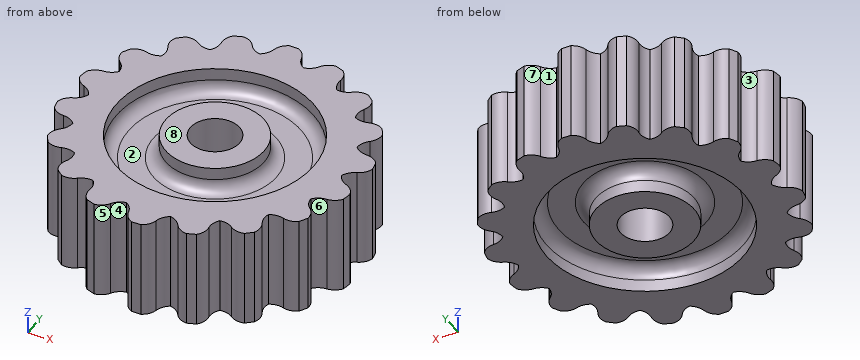
from build123d import *

# Parameters (mm, degrees)
CUT_EXTRUDE4_DEPTH      = 60.56828015
CUT_EXTRUDE4_DEPTH_BACK = 60.56828015


with BuildPart() as part:
    # Sketch1 → Revolve1 (revolve)
    with BuildSketch(Plane(origin=(0, 0, 0), x_dir=(0, 0, -1), z_dir=(1, 0, 0)), mode=Mode.PRIVATE) as revolve1_sk:
        with BuildLine():
            ThreePointArc((9.525, 25.4), (7.27993597, 24.47006403), (6.35, 22.225))
            Line((6.35, 22.225), (6.35, 15.875))
            ThreePointArc((6.35, 15.875), (7.27993597, 13.62993597), (9.525, 12.7))
            Line((9.525, 12.7), (12.7, 12.7))
            Line((12.7, 12.7), (12.7, 6.35))
            Line((12.7, 6.35), (-12.7, 6.35))
            Line((-12.7, 6.35), (-12.7, 12.7))
            Line((-12.7, 12.7), (-9.525, 12.7))
            ThreePointArc((-9.525, 12.7), (-7.27993597, 13.62993597), (-6.35, 15.875))
            Line((-6.35, 15.875), (-6.35, 22.225))
            ThreePointArc((-6.35, 22.225), (-7.27993597, 24.47006403), (-9.525, 25.4))
            Line((-9.525, 25.4), (-12.7, 25.4))
            Line((-12.7, 25.4), (-12.7, 38.1))
            Line((-12.7, 38.1), (12.7, 38.1))
            Line((12.7, 38.1), (12.7, 25.4))
            Line((12.7, 25.4), (9.525, 25.4))
        make_face()
    revolve(revolve1_sk.sketch.rotate(Axis((0, 0, 45.501840491), (0, 0, -1)), 90), axis=Axis((0, 0, 45.501840491), (0, 0, -1)))

    # Sketch2 → Cut-Extrude4 (cut, two sides: drawn at the far end of the back side and taken through both)
    with BuildSketch(Plane.XY.offset(12.7).offset(-CUT_EXTRUDE4_DEPTH_BACK)):
        with BuildLine():
            ThreePointArc((35.210604435, 2.593640551), (33.661156199, 1.568112092), (32.6644, 0))
            ThreePointArc((32.6644, 0), (33.661156199, -1.568112092), (35.210604435, -2.593640551))
            ThreePointArc((35.210604435, -2.593640551), (36.804464445, -3.712859333), (37.710053333, -5.437083557))
            ThreePointArc((37.710053333, -5.437083557), (38.1, 0), (37.710053333, 5.437083557))
            ThreePointArc((37.710053333, 5.437083557), (36.804464445, 3.712859333), (35.210604435, 2.593640551))
        make_face()
        with BuildLine():
            ThreePointArc((32.200067848, 14.479960862), (31.094814165, 12.98633683), (30.694495642, 11.17188277))
            ThreePointArc((30.694495642, 11.17188277), (32.16746601, 10.039250106), (33.974222474, 9.605511089))
            ThreePointArc((33.974222474, 9.605511089), (35.854756332, 9.098921688), (37.295450944, 7.788410548))
            ThreePointArc((37.295450944, 7.788410548), (35.802288852, 13.030967461), (33.576266749, 18.006785143))
            ThreePointArc((33.576266749, 18.006785143), (33.31501097, 16.076814721), (32.200067848, 14.479960862))
        make_face()
        with BuildLine():
            ThreePointArc((33.974222474, -9.605511089), (32.16746601, -10.039250106), (30.694495642, -11.17188277))
            ThreePointArc((30.694495642, -11.17188277), (31.094814165, -12.98633683), (32.200067848, -14.479960862))
            ThreePointArc((32.200067848, -14.479960862), (33.31501097, -16.076814721), (33.576266749, -18.006785143))
            ThreePointArc((33.576266749, -18.006785143), (35.802288852, -13.030967461), (37.295450944, -7.788410548))
            ThreePointArc((37.295450944, -7.788410548), (35.854756332, -9.098921688), (33.974222474, -9.605511089))
        make_face()
        with BuildLine():
            ThreePointArc((25.305727856, 24.619784192), (24.777978632, 22.838217687), (25.022382108, 20.996271598))
            ThreePointArc((25.022382108, 20.996271598), (26.793904679, 20.435730578), (28.640047877, 20.646096329))
            ThreePointArc((28.640047877, 20.646096329), (30.580435445, 20.813238467), (32.382466749, 20.074507397))
            ThreePointArc((32.382466749, 20.074507397), (29.186293283, 24.490207929), (25.392686862, 28.404602689))
            ThreePointArc((25.392686862, 28.404602689), (25.807275495, 26.501668986), (25.305727856, 24.619784192))
        make_face()
        with BuildLine():
            ThreePointArc((28.640047877, -20.646096329), (26.793904679, -20.435730578), (25.022382108, -20.996271598))
            ThreePointArc((25.022382108, -20.996271598), (24.777978632, -22.838217687), (25.305727856, -24.619784192))
            ThreePointArc((25.305727856, -24.619784192), (25.807275495, -26.501668986), (25.392686862, -28.404602689))
            ThreePointArc((25.392686862, -28.404602689), (29.186293283, -24.490207929), (32.382466749, -20.074507397))
            ThreePointArc((32.382466749, -20.074507397), (30.580435445, -20.813238467), (28.640047877, -20.646096329))
        make_face()
        with BuildLine():
            ThreePointArc((15.359143612, 31.790098199), (15.472553192, 29.935472436), (16.3322, 28.288200199))
            ThreePointArc((16.3322, 28.288200199), (18.188603008, 28.367360343), (19.851460823, 29.196457648))
            ThreePointArc((19.851460823, 29.196457648), (21.617662725, 30.017171516), (23.56367915, 29.939322386))
            ThreePointArc((23.56367915, 29.939322386), (19.05, 32.995567884), (14.146374183, 35.376405943))
            ThreePointArc((14.146374183, 35.376405943), (15.18680172, 33.730030848), (15.359143612, 31.790098199))
        make_face()
        with BuildLine():
            ThreePointArc((19.851460823, -29.196457648), (18.188603008, -28.367360343), (16.3322, -28.288200199))
            ThreePointArc((16.3322, -28.288200199), (15.472553192, -29.935472436), (15.359143612, -31.790098199))
            ThreePointArc((15.359143612, -31.790098199), (15.18680172, -33.730030848), (14.146374183, -35.376405943))
            ThreePointArc((14.146374183, -35.376405943), (19.05, -32.995567884), (23.56367915, -29.939322386))
            ThreePointArc((23.56367915, -29.939322386), (21.617662725, -30.017171516), (19.851460823, -29.196457648))
        make_face()
        with BuildLine():
            ThreePointArc((3.560019972, 35.126057191), (4.300909486, 33.422067408), (5.672113535, 32.168154367))
            ThreePointArc((5.672113535, 32.168154367), (7.389487378, 32.877467793), (8.668494618, 34.225295281))
            ThreePointArc((8.668494618, 34.225295281), (10.047480837, 35.600590674), (11.902764082, 36.193013237))
            ThreePointArc((11.902764082, 36.193013237), (6.615995569, 37.52117539), (1.1938, 38.081292541))
            ThreePointArc((1.1938, 38.081292541), (2.734575524, 36.890053188), (3.560019972, 35.126057191))
        make_face()
        with BuildLine():
            ThreePointArc((8.668494618, -34.225295281), (7.389487378, -32.877467793), (5.672113535, -32.168154367))
            ThreePointArc((5.672113535, -32.168154367), (4.300909486, -33.422067408), (3.560019972, -35.126057191))
            ThreePointArc((3.560019972, -35.126057191), (2.734575524, -36.890053188), (1.1938, -38.081292541))
            ThreePointArc((1.1938, -38.081292541), (6.615995569, -37.52117539), (11.902764082, -36.193013237))
            ThreePointArc((11.902764082, -36.193013237), (10.047480837, -35.600590674), (8.668494618, -34.225295281))
        make_face()
        with BuildLine():
            ThreePointArc((-8.668494618, 34.225295281), (-7.389487378, 32.877467793), (-5.672113535, 32.168154367))
            ThreePointArc((-5.672113535, 32.168154367), (-4.300909486, 33.422067408), (-3.560019972, 35.126057191))
            ThreePointArc((-3.560019972, 35.126057191), (-2.734575524, 36.890053188), (-1.1938, 38.081292541))
            ThreePointArc((-1.1938, 38.081292541), (-6.615995569, 37.52117539), (-11.902764082, 36.193013237))
            ThreePointArc((-11.902764082, 36.193013237), (-10.047480837, 35.600590674), (-8.668494618, 34.225295281))
        make_face()
        with BuildLine():
            ThreePointArc((-3.560019972, -35.126057191), (-4.300909486, -33.422067408), (-5.672113535, -32.168154367))
            ThreePointArc((-5.672113535, -32.168154367), (-7.389487378, -32.877467793), (-8.668494618, -34.225295281))
            ThreePointArc((-8.668494618, -34.225295281), (-10.047480837, -35.600590674), (-11.902764082, -36.193013237))
            ThreePointArc((-11.902764082, -36.193013237), (-6.615995569, -37.52117539), (-1.1938, -38.081292541))
            ThreePointArc((-1.1938, -38.081292541), (-2.734575524, -36.890053188), (-3.560019972, -35.126057191))
        make_face()
        with BuildLine():
            ThreePointArc((-19.851460823, 29.196457648), (-18.188603008, 28.367360343), (-16.3322, 28.288200199))
            ThreePointArc((-16.3322, 28.288200199), (-15.472553192, 29.935472436), (-15.359143612, 31.790098199))
            ThreePointArc((-15.359143612, 31.790098199), (-15.18680172, 33.730030848), (-14.146374183, 35.376405943))
            ThreePointArc((-14.146374183, 35.376405943), (-19.05, 32.995567884), (-23.56367915, 29.939322386))
            ThreePointArc((-23.56367915, 29.939322386), (-21.617662725, 30.017171516), (-19.851460823, 29.196457648))
        make_face()
        with BuildLine():
            ThreePointArc((-15.359143612, -31.790098199), (-15.472553192, -29.935472436), (-16.3322, -28.288200199))
            ThreePointArc((-16.3322, -28.288200199), (-18.188603008, -28.367360343), (-19.851460823, -29.196457648))
            ThreePointArc((-19.851460823, -29.196457648), (-21.617662725, -30.017171516), (-23.56367915, -29.939322386))
            ThreePointArc((-23.56367915, -29.939322386), (-19.05, -32.995567884), (-14.146374183, -35.376405943))
            ThreePointArc((-14.146374183, -35.376405943), (-15.18680172, -33.730030848), (-15.359143612, -31.790098199))
        make_face()
        with BuildLine():
            ThreePointArc((-28.640047877, 20.646096329), (-26.793904679, 20.435730578), (-25.022382108, 20.996271598))
            ThreePointArc((-25.022382108, 20.996271598), (-24.777978632, 22.838217687), (-25.305727856, 24.619784192))
            ThreePointArc((-25.305727856, 24.619784192), (-25.807275495, 26.501668986), (-25.392686862, 28.404602689))
            ThreePointArc((-25.392686862, 28.404602689), (-29.186293283, 24.490207929), (-32.382466749, 20.074507397))
            ThreePointArc((-32.382466749, 20.074507397), (-30.580435445, 20.813238467), (-28.640047877, 20.646096329))
        make_face()
        with BuildLine():
            ThreePointArc((-25.305727856, -24.619784192), (-24.777978632, -22.838217687), (-25.022382108, -20.996271598))
            ThreePointArc((-25.022382108, -20.996271598), (-26.793904679, -20.435730578), (-28.640047877, -20.646096329))
            ThreePointArc((-28.640047877, -20.646096329), (-30.580435445, -20.813238467), (-32.382466749, -20.074507397))
            ThreePointArc((-32.382466749, -20.074507397), (-29.186293283, -24.490207929), (-25.392686862, -28.404602689))
            ThreePointArc((-25.392686862, -28.404602689), (-25.807275495, -26.501668986), (-25.305727856, -24.619784192))
        make_face()
        with BuildLine():
            ThreePointArc((-33.974222474, 9.605511089), (-32.16746601, 10.039250106), (-30.694495642, 11.17188277))
            ThreePointArc((-30.694495642, 11.17188277), (-31.094814165, 12.98633683), (-32.200067848, 14.479960862))
            ThreePointArc((-32.200067848, 14.479960862), (-33.31501097, 16.076814721), (-33.576266749, 18.006785143))
            ThreePointArc((-33.576266749, 18.006785143), (-35.802288852, 13.030967461), (-37.295450944, 7.788410548))
            ThreePointArc((-37.295450944, 7.788410548), (-35.854756332, 9.098921688), (-33.974222474, 9.605511089))
        make_face()
        with BuildLine():
            ThreePointArc((-32.200067848, -14.479960862), (-31.094814165, -12.98633683), (-30.694495642, -11.17188277))
            ThreePointArc((-30.694495642, -11.17188277), (-32.16746601, -10.039250106), (-33.974222474, -9.605511089))
            ThreePointArc((-33.974222474, -9.605511089), (-35.854756332, -9.098921688), (-37.295450944, -7.788410548))
            ThreePointArc((-37.295450944, -7.788410548), (-35.802288852, -13.030967461), (-33.576266749, -18.006785143))
            ThreePointArc((-33.576266749, -18.006785143), (-33.31501097, -16.076814721), (-32.200067848, -14.479960862))
        make_face()
        with BuildLine():
            ThreePointArc((-35.210604435, -2.593640551), (-33.661156199, -1.568112092), (-32.6644, 0))
            ThreePointArc((-32.6644, 0), (-33.661156199, 1.568112092), (-35.210604435, 2.593640551))
            ThreePointArc((-35.210604435, 2.593640551), (-36.804464445, 3.712859333), (-37.710053333, 5.437083557))
            ThreePointArc((-37.710053333, 5.437083557), (-38.1, 0), (-37.710053333, -5.437083557))
            ThreePointArc((-37.710053333, -5.437083557), (-36.804464445, -3.712859333), (-35.210604435, -2.593640551))
        make_face()
    extrude(amount=CUT_EXTRUDE4_DEPTH + CUT_EXTRUDE4_DEPTH_BACK, mode=Mode.SUBTRACT)


solid = part.part
Geometry check sheet. Reference: the model listing, model coordinates, mm. Face numbers are marked on the shaded views. A direction names the side the tool comes from. Round coordinates to 2 decimals unless told otherwise and drop trailing zeros. Answer in a Markdown table with one row per item. Add a question column.
Item 1: Material ranges on L1, parallel to Y at x = 0, z = -10.6; L2, parallel to X at y = 29.5, z = 0; L3, parallel to Y at x = -8.5, z = -11, recorded low to high. Write a range as [from, to].
Item 2: Draft check along Y on the marked faces 5, 6, 7 and 8. Enter one of: released by +Y, released by -Y, zero draft, split by the parting line, or undercut.
Item 3: Set-up check for the marked faces 1, 2, 3 and 4: record each of +Z, -Z, +X, -X, +Y, -Y from which the full face is reachable in a straight line by a thin tool's end or side.
Item 4: Depth check by flat-ended pin: pin 1 Ø5 at (x, y) = (-1, -17) entering from +Z; pin 2 Ø1.5 at (x, z) = (-9, -7) entering from -Y; pin 3 Ø11.5 at (x, y) = (0, 0) entering from -Z; pin 4 Ø1.5 at (y, z) = (24.5, 6) entering from +X. Enter the tip coordinate at first touch or a pass-through.
Filled in:
| question | item | result |
|---|---|---|
| 1 | L1 | y = [-38.1, -25.4], [-12.7, -6.35], [6.35, 12.7], [25.4, 38.1] |
| 1 | L2 | x = [-24.11, -20.29], [-15.62, 15.62], [20.29, 24.11] |
| 1 | L3 | y = [-33.97, -23.94], [-9.44, 9.44], [23.94, 33.97] |
| 2 | face 5 | released by -Y |
| 2 | face 6 | undercut |
| 2 | face 7 | released by +Y |
| 2 | face 8 | zero draft |
| 3 | face 1 | +Z, -Z, +Y |
| 3 | face 2 | +Z |
| 3 | face 3 | +Z, -Z, -X |
| 3 | face 4 | +Z, -Z, -Y |
| 4 | pin 1 | stops at z = 6.65 |
| 4 | pin 2 | stops at y = -35.4 |
| 4 | pin 3 | passes through |
| 4 | pin 4 | stops at x = 25.58 |
